Design review of the part built by this model. Coordinates are the model's own, in mm. A direction names the side the tool comes from. Coordinates: 2 decimals unless noted, no trailing zeros. Use CSV: the item, a comma, the result in double quotes.
```python
from build123d import *

# Parameters (mm, degrees)
F0_R     = 2
F0_R_2   = 2.5
F1_DEPTH = 2
F2_SIZE  = 1.99999
F3_R     = 4
F3_R_2   = 2.5
F4_DEPTH = 9


# Not quite as in the source:
# - a fillet or chamfer is up to 0.001 mm smaller than in the source, because OpenCascade refuses the exact size


with BuildPart() as f1:
    # F0 (on Front) → F1 (new body)
    with BuildSketch(Plane.XZ):
        with BuildLine():
            Line((-10.6066017178, -3.5355339059), (-3.5355339059, -10.6066017178))
            ThreePointArc((-3.5355339059, -10.6066017178), (0, -12.0710678119), (3.5355339059, -10.6066017178))
            Line((3.5355339059, -10.6066017178), (10.6066017178, -3.5355339059))
            ThreePointArc((10.6066017178, -3.5355339059), (12.0710678119, 0), (10.6066017178, 3.5355339059))
            Line((10.6066017178, 3.5355339059), (3.5355339059, 10.6066017178))
            ThreePointArc((3.5355339059, 10.6066017178), (0, 12.0710678119), (-3.5355339059, 10.6066017178))
            Line((-3.5355339059, 10.6066017178), (-10.6066017178, 3.5355339059))
            ThreePointArc((-10.6066017178, 3.5355339059), (-12.0710678119, 0), (-10.6066017178, -3.5355339059))
        make_face()
        with Locations((-7, 0)):
            Circle(F0_R, mode=Mode.SUBTRACT)
        with Locations((0, -7)):
            Circle(F0_R, mode=Mode.SUBTRACT)
        Circle(F0_R_2, mode=Mode.SUBTRACT)
        with Locations((7, 0)):
            Circle(F0_R, mode=Mode.SUBTRACT)
        with Locations((0, 7)):
            Circle(F0_R, mode=Mode.SUBTRACT)
    extrude(amount=F1_DEPTH)

    # F2 (size 2 in the source; OpenCascade refuses exactly that, so slightly less here)
    f2_edges = [f1.edges().sort_by_distance(p)[0] for p in [
        (5, -2, 0),
        (-2, -2, -7),
        (-9, -2, 0),
        (-2, -2, 7),
    ]]
    chamfer(f2_edges, length=F2_SIZE)

    # F3 (on face) → F4 (join)
    with BuildSketch(Plane(origin=(0, 0, 0), x_dir=(-1, 0, 0), z_dir=(0, 1, 0))):
        Circle(F3_R)
        Circle(F3_R_2, mode=Mode.SUBTRACT)
    extrude(amount=F4_DEPTH)


solid = f1.part
```
Item 1: Clearance check with flat-ended pins moving along their axes: pin 1 (1.5 mm diameter, centred on x = -7.5, z = 6.5, fed in from +Y); pin 2 (6 mm diameter, centred on y = 5.5, z = -3.5, fed in from +X). State where each tip first meets the part, or that it passes through.
Checked values:
pin 1,"y = 0"
pin 2,"x = 3.97"
Item 2: To check wall thickness, follow line 1 along Z through (x, y) = (-1.25, -1); line 2 along Y through (x, z) = (-3.75, 3); line 3 along X through (y, z) = (4, 1.5). State the ranges of each line that lie inside material, in increasing order.
Checked values:
line 1,"-11.91 to -9.73, -4.27 to -2.17, 2.17 to 4.27, 9.73 to 11.91"
line 2,"-2 to 0"
line 3,"-3.71 to -2, 2 to 3.71"
Item 3: Machinability: for faces 1 (the face through (-0.05, -0.99, -12.07)), 2 (the face through (0.867, 4.437, -3.905)), which of the approach directions +Z, -Z, +X, -X, +Y, -Y give a long, thin tool a straight path to every point of the face, cutting with its end or side? Answer none if there is none.
Checked values:
face 1,"-Z, +Y, -Y"
face 2,"+Y"
Item 4: Add section A-A (z = 0). State how many separate pieces and enclosed holes the cut face has, then the cut area to 3 significant figures.
Checked values:
separate pieces,"4"
enclosed holes,"0"
area,"41.3 mm^2"
